Verification items for the finished model (mm, model axes). A direction names the side the tool comes from. Give positions to 0.01 mm unless a question says otherwise; leave off trailing zeros. Loops run counter-clockwise (first coordinate to the right, second up) from the corner with the lowest first, then second, coordinate; pieces in that order, holes last. Notation, with made-up numbers: (-18, 5.5) - (0, 5.5) arc R24 cw to (0, 33.5) - close; hole circle Ø11 at (13, 31.25). An arc over 180 degrees is marked (long way). One line per item, written item: value. Start each with the question number.
1. Sectioned sample at C-C (y = 33). Record the cut outline in (x, z).
2. Scan lines: L1, parallel to Y at x = 11.5, z = -18.25; L2, parallel to Y at x = 48, z = -12.5; L3, parallel to X at y = 91, z = -17. Record each from-to range of solid material in increasing order. Write a range as [from, to].
3. Gauge pin test, flat ends, axial feed: pin 1 (6 mm diameter, centred on x = 51, z = -16.5, fed in from +Y); pin 2 (5 mm diameter, centred on y = 84, z = -3, fed in from +X); pin 3 (1.5 mm diameter, centred on y = 79, z = -11.5, fed in from -X). Record the tip position at first contact, or that the pin passes through.
4. Mould release check, pull along X, two halves, no side actions. Record for faces 3 (the flat face through (65, 42, -20)), 4 (the flat face through (0, 1, -10)), 5 (the cylindrical face through (50.17, 13.35, -10.14)): pulls with the +X half, pulls with the -X half, needs draft (parallel to the pull), parting line crosses it, or undercut.
5. Sectioned sample at B-B (x = 9.5). Record the cut outline in (y, z), plus the area to 3 significant figures.
6. Access from +Z, -Z, +X, -X, +Y, -Y to the whole of each face (thin tool, end or side, straight path). Record for faces 1 (the flat face through (8, 3, -10)), 2 (the flat face through (65, 46, 0)).
7. Sectioned sample at A-A (z = -11.75). Record the cut outline in (x, y).
Autodesk Inventor part; units mm, degrees
ref_plane "YZ Plane" through (0, 0, 0) normal (1, 0, 0) x (0, 1, 0)
ref_plane "XZ Plane" through (0, 0, 0) normal (0, 1, 0) x (-1, 0, 0)
ref_plane "XY Plane" through (0, 0, 0) normal (0, 0, 1) x (1, 0, 0)
sketch "Sketch2" plane through (0, 0, 0) normal (0, 1, 0) x (-1, 0, 0)
  line L0 (0, 0) -> (-160, 0)
  line L1 (-160, 0) -> (-160, -20)
  line L2 (-160, -20) -> (0, -20)
  line L3 (0, -20) -> (0, 0)
  dimension "d0" = 160
  dimension "d1" = 20
extrude "Extrusion1" add sketch "Sketch2" along normal blind 3
sketch "Sketch3" plane through (0, 3, 0) normal (0, 1, 0) x (1, 0, 0)
  line L0 (160, 20) -> (0, 20)
  line L1 (160, 0) -> (160, 20)
  line L2 (160, 20) -> (160, 0)
  line L3 (15, 20) -> (15, 0)
  line L4 (0, 0) -> (160, 0)
  line L5 (0, 20) -> (0, 0)
  dimension "d8" = 15
bend part "Bend Part1" radius 50 angle 82 line through (15, 3, -20) along (0, 0, 1) centre toward (0, 1, 0) moving side (1, 0, 0) both sides no
properties part number "ball-reload-left"
Results are:
1. outline: (60.83, -20) - (64.08, -20) - (64.08, 0) - (60.83, 0) - close
2. L1: y = [0, 3]
2. L2: y = [11.53, 15.44]
2. L3: x = [70.83, 73.86]
3. pin 1: stops at y = 21.71
3. pin 2: stops at x = 73.23
3. pin 3: stops at x = 69.04
4. face 3: needs draft
4. face 4: pulls with the -X half
4. face 5: pulls with the +X half
5. outline: (0, -20) - (3, -20) - (3, 0) - (0, 0) - close
5. area: 60.0 mm^2
6. face 1: +Z, -Z, -X, +Y
6. face 2: +Z, +X, -X, +Y, -Y
7. outline: (0, 0) - (15, 0) arc R53 ccw to (67.48, 45.62) - (77.71, 118.35) - (74.73, 118.77) - (64.51, 46.04) arc R50 cw to (15, 3) - (0, 3) - close
